The model under review builds one solid part; all positions refer to its coordinate system, in mm. Coordinates: 2 decimals unless noted, no trailing zeros. Write each loop counter-clockwise with the first axis right and the second up, starting at its lowest first coordinate (ties: lowest second). Pieces come first, ordered by that corner, then holes. Notation, with made-up numbers: (50, -34.5) -> (61, -34.5) arc R36 cw to (61, 4.5) -> close; hole circle Ø5 at (-5, 51.25). An arc over 180 degrees is marked (long way). Put each result on its own line as item: value. Start each with the question number.
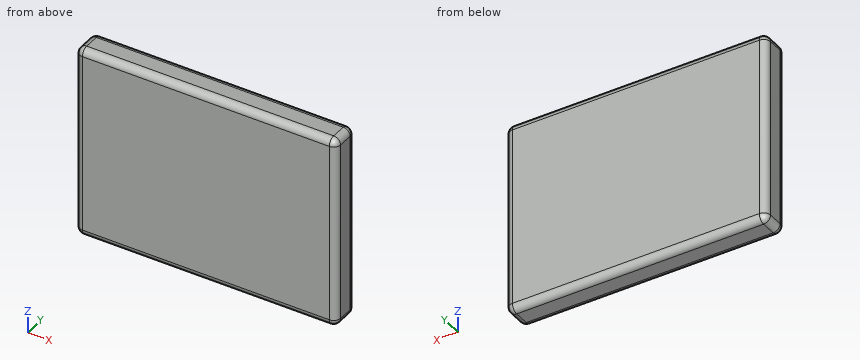
from build123d import *

# Parameters (mm, degrees)
F0_W     = 1900
F0_H     = 1400
F1_DEPTH = 105
F2_R     = 50
F3_R     = 50


with BuildPart() as f1:
    # F0 (on Front) → F1 (new body, symmetric)
    with BuildSketch(Plane.XZ):
        with Locations((-50, 0)):
            Rectangle(F0_W, F0_H)
    extrude(amount=F1_DEPTH, both=True)

    # F2
    f2_edges = [f1.edges().sort_by_distance(p)[0] for p in [
        (-1000, 0, 700),
        (900, 0, 700),
        (900, 0, -700),
        (-1000, 0, -700),
    ]]
    fillet(f2_edges, radius=F2_R)

    # F3
    f3_edges = [f1.edges().sort_by_distance(p)[0] for p in [
        (-50, -105, 700),
        (885.355339, -105, 685.355339),
        (-985.355339, -105, 685.355339),
        (900, -105, 0),
        (-1000, -105, 0),
        (885.355339, -105, -685.355339),
        (-985.355339, -105, -685.355339),
        (-50, -105, -700),
        (-50, 105, 700),
        (885.355339, 105, 685.355339),
        (-985.355339, 105, 685.355339),
        (900, 105, 0),
        (-1000, 105, 0),
        (885.355339, 105, -685.355339),
        (-985.355339, 105, -685.355339),
        (-50, 105, -700),
    ]]
    fillet(f3_edges, radius=F3_R)


solid = f1.part
1. Consider section A-A on y = -81.5. State the section outline as (x, z) points, then the cut area to 3 significant figures.
2. Wall thickness on line 1 (X direction, y = 56.5, z = -486); line 2 (X direction, y = 57.5, z = -419.5); line 3 (Z direction, x = -788, y = 60): over which ranges is each line inside the solid? List them lowest first. Write a range as from..to.
3. Insertion check: P1, Ø8, axis at y = 62, z = 141.5, coming from the +X side. The pin has a flat end and moves straight along its axis. Give the tip position at first contact, or say it passes through.
4. Consider section B-B on y = 79.5. State the section outline as (x, z) points, then the cut area to 3 significant figures.
Output values:
1. outline: (-992.4, -650) arc R42.4 ccw to (-950, -692.4) -> (850, -692.4) arc R42.4 ccw to (892.4, -650) -> (892.4, 650) arc R42.4 ccw to (850, 692.4) -> (-950, 692.4) arc R42.4 ccw to (-992.4, 650) -> close
1. area: 2,610,000 mm^2
2. line 1: x = -999.98..899.98
2. line 2: x = -999.94..899.94
2. line 3: z = -699.75..699.75
3. P1: stops at x = 899.91
4. outline: (-993.59, -650) arc R43.59 ccw to (-950, -693.59) -> (850, -693.59) arc R43.59 ccw to (893.59, -650) -> (893.59, 650) arc R43.59 ccw to (850, 693.59) -> (-950, 693.59) arc R43.59 ccw to (-993.59, 650) -> close
4. area: 2,620,000 mm^2
